Can you work these out from the model? Positions are in its coordinate system, mm. Give positions to 0.01 mm unless a question says otherwise; leave off trailing zeros. Write each loop counter-clockwise with the first axis right and the second up, starting at its lowest first coordinate (ties: lowest second). Pieces come first, ordered by that corner, then holes. Notation, with made-up numbers: (-32.5, -3) -> (7.5, -3) arc R9 ccw to (7.5, 2) -> close; hole circle Ø8 at (61, -36). An arc over 180 degrees is marked (long way). One line per item, written item: value.
from build123d import *

# Parameters (mm, degrees)
SKETCH1_W           = 20
SKETCH1_H           = 30
BOSS_EXTRUDE1_DEPTH = 5
SKETCH2_R           = 2
CUT_EXTRUDE1_DEPTH  = 5
SKETCH3_W           = 20
SKETCH3_H           = 5
BOSS_EXTRUDE2_DEPTH = 7
SKETCH4_W           = 20
SKETCH4_H           = 5
BOSS_EXTRUDE3_DEPTH = 30
SKETCH5_R           = 2
CUT_EXTRUDE2_DEPTH  = 7


with BuildPart() as part:
    # Sketch1 → Boss-Extrude1 (new body)
    with BuildSketch(Plane.XY):
        Rectangle(SKETCH1_W, SKETCH1_H)
    extrude(amount=BOSS_EXTRUDE1_DEPTH)

    # Sketch2 → Cut-Extrude1 (cut)
    with BuildSketch(Plane.XY.offset(5)):
        with Locations((0, 7.5)):
            Circle(SKETCH2_R)
        with Locations((0, -7.5)):
            Circle(SKETCH2_R)
    extrude(amount=-CUT_EXTRUDE1_DEPTH, mode=Mode.SUBTRACT)

    # Sketch3 → Boss-Extrude2 (add)
    with BuildSketch(Plane.XZ.offset(15)):
        with Locations((0, 2.5)):
            Rectangle(SKETCH3_W, SKETCH3_H)
    extrude(amount=BOSS_EXTRUDE2_DEPTH)

    # Sketch4 → Boss-Extrude3 (add)
    with BuildSketch(Plane(origin=(0, 15, 0), x_dir=(1, 0, 0), z_dir=(0, 1, 0))):
        with Locations((0, -2.5)):
            Rectangle(SKETCH4_W, SKETCH4_H)
    extrude(amount=BOSS_EXTRUDE3_DEPTH)

    # Sketch5 → Cut-Extrude2 (cut)
    with BuildSketch(Plane(origin=(0, 0, 0), x_dir=(-1, 0, 0), z_dir=(0, 0, -1))):
        with Locations((0, 22.5)):
            Circle(SKETCH5_R)
    extrude(amount=-CUT_EXTRUDE2_DEPTH, mode=Mode.SUBTRACT)


solid = part.part
1) If we section it at B-B (z = 1.2): Write out the boundary of the cut face in (x, y).
Answer list:
outline: (-10, -22) -> (10, -22) -> (10, 45) -> (-10, 45) -> close; hole circle Ø4 at (0, -7.5); hole circle Ø4 at (0, 7.5); hole circle Ø4 at (0, 22.5)
2) If we section it at C-C (y = -7.5): Write out the boundary of the cut face in (x, z).
Answer list:
outline: (-10, 0) -> (-2, 0) -> (-2, 5) -> (-10, 5) -> close; (2, 0) -> (10, 0) -> (10, 5) -> (2, 5) -> close
3) If we section it at A-A (x = 0): Write out the boundary of the cut face in (y, z), and give its area (3 significant figures).
Answer list:
outline: (-22, 0) -> (-9.5, 0) -> (-9.5, 5) -> (-22, 5) -> close; (-5.5, 0) -> (5.5, 0) -> (5.5, 5) -> (-5.5, 5) -> close; (9.5, 0) -> (20.5, 0) -> (20.5, 5) -> (9.5, 5) -> close; (24.5, 0) -> (45, 0) -> (45, 5) -> (24.5, 5) -> close
area: 275 mm^2
4) We'd pull the mould along Y, two halves only. Please class faces 1 (the face through (10, 11, 3)), 2 (the face through (-0.923, 20.726, 2.465)), 3 (the face through (0, -22, 3)): released by +Y, released by -Y, zero draft, split by the parting line, or undercut.
Answer list:
face 1: zero draft
face 2: undercut
face 3: released by -Y
5) Will these pins go through, and if not, where does the flat tip stop? pin 1 (3.5 mm diameter, centred on x = 0, y = 22.5, fed in from +Z); pin 2 (4.5 mm diameter, centred on x = 0, y = -7.5, fed in from +Z).
Answer list:
pin 1: passes through
pin 2: stops at z = 5
6) I need wall thicknesses on L1, parallel to Y at x = 0, z = 2.55; L2, parallel to Y at x = -1, z = 4.4; L3, parallel to X at y = 21.5, z = 1.25. Which ranges of each line are inside material? Lowest first, please.
Answer list:
L1: y = -22 to -9.5, -5.5 to 5.5, 9.5 to 20.5, 24.5 to 45
L2: y = -22 to -9.23, -5.77 to 5.77, 9.23 to 20.77, 24.23 to 45
L3: x = -10 to -1.73, 1.73 to 10
